Autodesk Inventor part; units mm, degrees
ref_plane "Work Plane1" through (0, 0, 7) normal (0, 0, -1) x (-1, 0, 0)
ref_plane "YZ Plane" through (0, 0, 0) normal (1, 0, 0) x (0, 1, 0)
ref_plane "XZ Plane" through (0, 0, 0) normal (0, 1, 0) x (-1, 0, 0)
sketch "Sketch1" plane through (0, 0, 0) normal (0, 0, 1) x (1, 0, 0)
  circle A0 centre (0, 0) radius 12.15
  dimension "d0" = 24.3
extrude "Extrusion1" add sketch "Sketch1" along normal blind 17
sketch "Sketch2" plane through (0, 0, 17) normal (0, 0, 1) x (1, 0, 0)
  circle A0 centre (0, 0) radius 11.15
  dimension "d3" = 22.3
extrude "Extrusion2" cut sketch "Sketch2" against normal blind 20
ref_plane "Work Plane1" through (0, 0, 7) normal (0, 0, -1) x (-1, 0, 0)
sketch "Sketch3" plane through (0, 0, 7) normal (0, 0, -1) x (-1, 0, 0)
  circle A0 centre (0, 0) radius 11.15
  circle A1 centre (0, 0) radius 9
  dimension "d7" = 18
extrude "Extrusion3" add sketch "Sketch3" against normal blind 2.8
properties part number "_3DPrint"
Model file for the job. Use its own axes, mm. A direction names the side the tool comes from. Round coordinates to 2 decimals unless told otherwise and drop trailing zeros. Write each loop counter-clockwise with the first axis right and the second up, starting at its lowest first coordinate (ties: lowest second). Pieces come first, ordered by that corner, then holes. Notation, with made-up numbers: (-10.5, -5.75) - (5.5, -5.75) arc R18 cw to (5.5, 17.25) - close; hole circle Ø10 at (53.25, 15). An arc over 180 degrees is marked (long way). Use CSV: the item, a comma, the result in double quotes. Start each with the question number.
Item 1: Pin check, flat tips, straight feed: P1, Ø3, axis at x = 3.5, y = -7, coming from the +Z side; P2, Ø5, axis at x = 1, z = 10, coming from the -Y side; P3, Ø1.5, axis at y = 8, z = 10, coming from the -X side; P4, Ø14.5, axis at x = 0, y = 0, coming from the -Z side. Stop position of each tip, or through.
Item 2: Band-saw the part on A-A (x = 0). Write the cut outline in (y, z), and give its area (3 significant figures).
Item 3: Band-saw the part on D-D (x = 10.25). Write the cut outline in (y, z), and give its area (3 significant figures).
Item 4: Drill centre lines: L1, parallel to Y at x = -0.25, z = 7.75; L2, parallel to Y at x = 0, z = 11.75; L3, parallel to Z at x = 8.5, y = 5. Where is each one in solid material? Low to high. Write a range as [from, to].
Item 5: Band-saw the part on C-C (z = 1.25). Write the cut outline in (x, y), and give its area (3 significant figures).
Item 6: Two-plate mould, pull along Y, no slides. Class faces 1 (the face through (1.172, 8.923, 8.38)), 2 (the face through (11, -4, 17)), 3 (the face through (-2.63, 11.86, 8.38)): released by +Y, released by -Y, zero draft, split by the parting line, or undercut.
Item 7: Tool access for faces 4 (the face through (11, -4, 0)), 5 (the face through (10.635, 3.349, 13.45)), 6 (the face through (-0.77, 9.14, 7)): list every direction of +Z, -Z, +X, -X, +Y, -Y with a clear straight run to the whole face (end or side of a thin tool).
Checked values:
1,P1,"stops at z = 9.8"
1,P2,"stops at y = -12.15"
1,P3,"stops at x = -9.75"
1,P4,"passes through"
2,outline,"(-12.15, 0) - (-11.15, 0) - (-11.15, 7) - (-9, 7) - (-9, 9.8) - (-11.15, 9.8) - (-11.15, 17) - (-12.15, 17) - close; (9, 7) - (11.15, 7) - (11.15, 0) - (12.15, 0) - (12.15, 17) - (11.15, 17) - (11.15, 9.8) - (9, 9.8) - close"
2,area,"46.0 mm²"
3,outline,"(-6.52, 0) - (-4.39, 0) - (-4.39, 7) - (4.39, 7) - (4.39, 0) - (6.52, 0) - (6.52, 17) - (4.39, 17) - (4.39, 9.8) - (-4.39, 9.8) - (-4.39, 17) - (-6.52, 17) - close"
3,area,"97.2 mm²"
4,L1,"y = [-12.15, -9], [9, 12.15]"
4,L2,"y = [-12.15, -11.15], [11.15, 12.15]"
4,L3,"z = [7, 9.8]"
5,outline,"circle Ø24.3 at (0, 0); hole circle Ø22.3 at (0, 0)"
5,area,"73.2 mm²"
6,face 1,"undercut"
6,face 2,"zero draft"
6,face 3,"split by the parting line"
7,face 4,"-Z, +X, -X, +Y, -Y"
7,face 5,"+Z"
7,face 6,"-Z"
